Part print with two shaded views. Sizes in mm from the minimum x, y, z corner. A direction names the side the tool comes from. Coordinates: 2 decimals unless noted, no trailing zeros. Loops run counter-clockwise (first coordinate to the right, second up) from the corner with the lowest first, then second, coordinate; pieces in that order, holes last. Notation, with made-up numbers: (11, -34.75) - (48, -34.75) arc R30 cw to (48, 0.25) - close; hole circle Ø9 at (-38, 65). An arc over 180 degrees is marked (long way). Write each question's results on one line, items separated by ' | '. Start each with the question number.
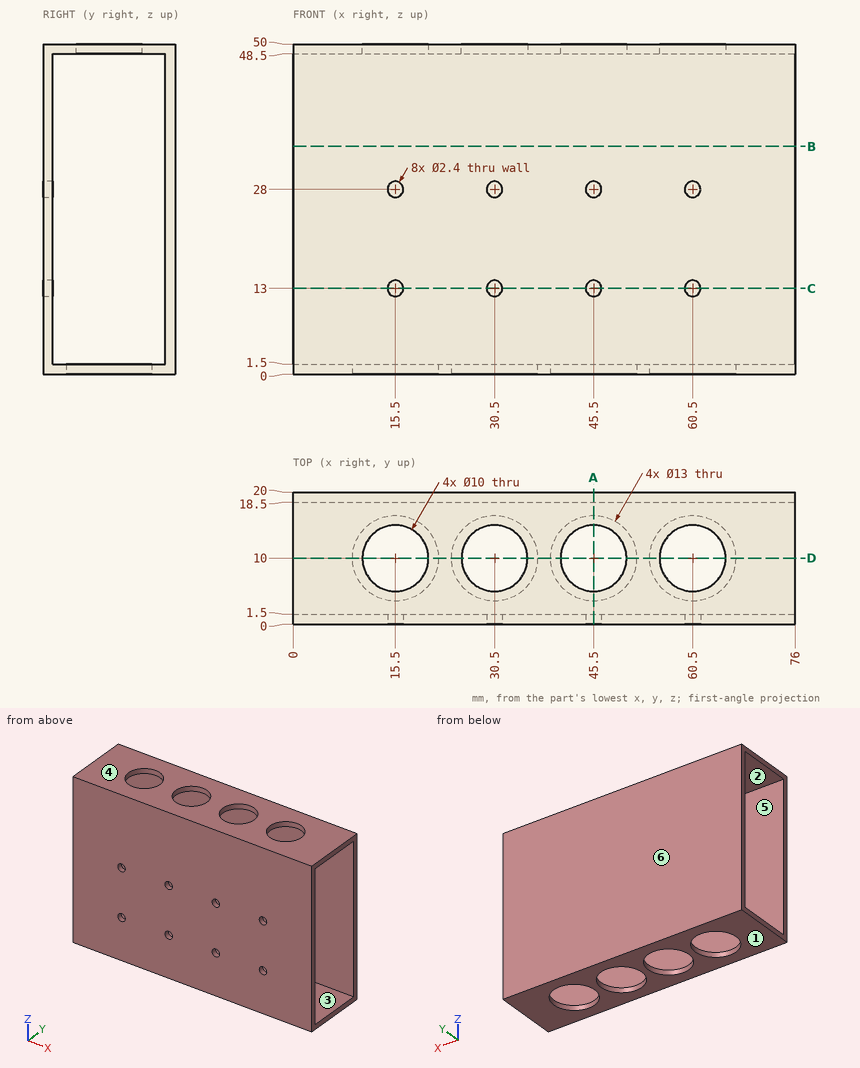
Q1. Mould opens along Z. For the marked faces 1, 2, 3 and 4 say: +Z half, -Z half, draft (parallel to the pull), parting line (faces both ways), or undercut.
Q2. Pin check, flat tip, straight feed: pin 1 (1.4 mm diameter, centred on x = 30.5, z = 28, fed in from -Y). Stop position of the tip, or through.
Q3. Cut at D-D (y = 10). State how many separate pieces and enclosed holes the cut face has, and give its area (3 significant figures).
Q4. Cut at A-A (x = 45.5). List the corners of the cut face in (y, z).
Q5. Which spindle directions (+Z, -Z, +X, -X, +Y, -Y) get a long thin tool onto all of the face, cutting with end or side? Do the marked faces 5 and 6. Say none if no direction does.
Q6. Cut at B-B (z = 34.5). List the corners of the cut face in (x, y).
Q7. Cut at C-C (z = 13). List the corners of the cut face in (x, y).
Q8. Drill centre lines: L1, parallel to Z at x = 45.5, y = 1.1; L2, parallel to Z at x = 71, y = 18; L3, parallel to X at y = 0.8, z = 13. Where is each one in solid material? Low to high. Write a range as from..to.
Check result:
1) face 1: -Z half | face 2: undercut | face 3: undercut | face 4: +Z half
2) pin 1: y = 18.5
3) separate pieces: 10 | enclosed holes: 0 | area: 90.0 mm²
4) outline: (0, 0) - (3.5, 0) - (3.5, 1.5) - (1.5, 1.5) - (1.5, 11.8) - (0, 11.8) - close; (0, 14.2) - (1.5, 14.2) - (1.5, 26.8) - (0, 26.8) - close; (0, 29.2) - (1.5, 29.2) - (1.5, 48.5) - (5, 48.5) - (5, 50) - (0, 50) - close; (15, 48.5) - (18.5, 48.5) - (18.5, 1.5) - (16.5, 1.5) - (16.5, 0) - (20, 0) - (20, 50) - (15, 50) - close
5) face 5: +X, -X | face 6: +Z, -Z, +X, -X, +Y
6) outline: (0, 0) - (76, 0) - (76, 1.5) - (0, 1.5) - close; (0, 18.5) - (76, 18.5) - (76, 20) - (0, 20) - close
7) outline: (0, 0) - (14.3, 0) - (14.3, 1.5) - (0, 1.5) - close; (0, 18.5) - (76, 18.5) - (76, 20) - (0, 20) - close; (16.7, 0) - (29.3, 0) - (29.3, 1.5) - (16.7, 1.5) - close; (31.7, 0) - (44.3, 0) - (44.3, 1.5) - (31.7, 1.5) - close; (46.7, 0) - (59.3, 0) - (59.3, 1.5) - (46.7, 1.5) - close; (61.7, 0) - (76, 0) - (76, 1.5) - (61.7, 1.5) - close
8) L1: 0..11.8, 14.2..26.8, 29.2..50 | L2: 0..1.5, 48.5..50 | L3: 0..14.3, 16.7..29.3, 31.7..44.3, 46.7..59.3, 61.7..76
